The listing builds one solid part. Answer for the finished solid, in the listing's coordinates (mm). Face numbers are marked on the shaded views. A direction names the side the tool comes from. Give positions to 0.01 mm unless a question says otherwise; leave off trailing zeros. Order: outer loops, then holes, each group sorted by start corner. A loop starts at its lowest first (then second) coordinate and runs counter-clockwise, first axis right, second up. Notation, with made-up numbers: (79, 76) - (93, 76) arc R11 ccw to (93, 97) - close; hole circle Ø2 at (-3.75, 59.25). An arc over 180 degrees is marked (long way). Answer in a Markdown table with one row per item.
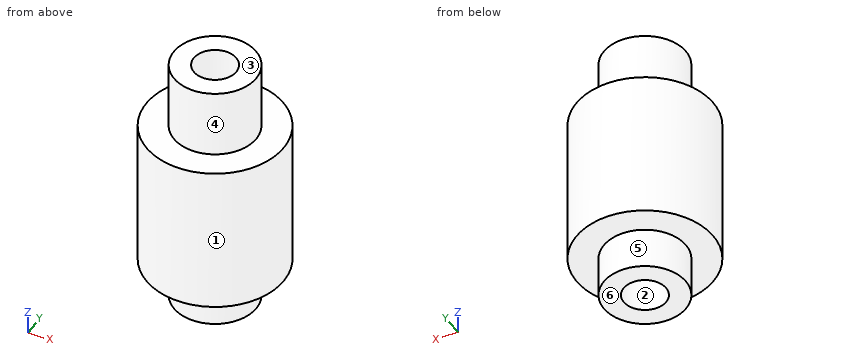
Autodesk Inventor part; units mm, degrees
ref_plane "YZ Plane" through (0, 0, 0) normal (1, 0, 0) x (0, 1, 0)
ref_plane "XZ Plane" through (0, 0, 0) normal (0, 1, 0) x (-1, 0, 0)
ref_plane "XY Plane" through (0, 0, 0) normal (0, 0, 1) x (1, 0, 0)
sketch "スケッチ1" plane through (0, 0, 0) normal (1, 0, 0) x (0, 1, 0)
  line L0 (0, 0) -> (3, 0)
  line L1 (3, 0) -> (3, 5)
  line L2 (3, 5) -> (0, 5)
  line L3 (0, 5) -> (0, 0)
  line L4 (0, 0) -> (5, 0)
  line L5 (5, 0) -> (5, -11)
  line L6 (5, -11) -> (0, -11)
  line L7 (0, -11) -> (0, 0)
  line L8 (0, -11) -> (3, -11)
  line L9 (3, -11) -> (3, -14)
  line L10 (3, -14) -> (0, -14)
  line L11 (0, -14) -> (0, -11)
  dimension "d0" = 3
  dimension "d1" = 5
  dimension "d2" = 5
  dimension "d3" = 11
  dimension "d4" = 3
  dimension "d5" = 3
revolve "回転1" add sketch "スケッチ1" angle 360 about axis through (0, 0, -11) along (0, 0, 1)
sketch "スケッチ2" plane through (0, 0, 5) normal (0, 0, 1) x (1, 0, 0)
  point P0 (0, 0)
  point P1 (0, 0)
hole "穴1" at (0, 0, 5) direction (0, 0, -1) diameter 3.1 end through all
properties part number "ベース板連結棒" material "アルミニウム 6061"
Item 1: Which of the six approach directions +Z, -Z, +X, -X, +Y, -Y give full straight-line access (tool end or side, diameter ignored) to the marked faces 4, 5 and 6?
Answer block:
| item | result |
|---|---|
| face 4 | +Z |
| face 5 | -Z |
| face 6 | -Z, +X, -X, +Y, -Y |
Item 2: Consider line 1 (Y direction, x = 0, z = -4.5); line 2 (Z direction, x = 4.75, y = -0.75). Determine where each line is inside the solid, lowest interval first.
Answer block:
| item | result |
|---|---|
| line 1 | -5 to -1.55, 1.55 to 5 |
| line 2 | -11 to 0 |
Item 3: This flat-tipped pin is pushed along its axis until it touches: P1, Ø1.5, axis at y = -1, z = -1.5, coming from the +X side. Where does it stop, or does it pass through?
Answer block:
| item | result |
|---|---|
| P1 | x = 4.99 |
Item 4: Determine the mould class of the marked faces 1, 2 and 3 for opening direction Y: pulls with the +Y half, pulls with the -Y half, needs draft (parallel to the pull), parting line crosses it, or undercut.
Answer block:
| item | result |
|---|---|
| face 1 | parting line crosses it |
| face 2 | undercut |
| face 3 | needs draft |
Item 5: Find section D-D on z = -10. Write down the section's boundary in (x, y).
Answer block:
| item | result |
|---|---|
| outline | circle Ø10 at (0, 0); hole circle Ø3.1 at (0, 0) |
Item 6: Find section C-C on x = 2. Write down the section's boundary in (y, z).
Answer block:
| item | result |
|---|---|
| outline | (-4.58, -11) - (-2.24, -11) - (-2.24, -14) - (2.24, -14) - (2.24, -11) - (4.58, -11) - (4.58, 0) - (2.24, 0) - (2.24, 5) - (-2.24, 5) - (-2.24, 0) - (-4.58, 0) - close |
Item 7: Find section A-A on y = 0. Write down the section's boundary in (x, z).
Answer block:
| item | result |
|---|---|
| outline | (-5, -11) - (-3, -11) - (-3, -14) - (-1.55, -14) - (-1.55, 5) - (-3, 5) - (-3, 0) - (-5, 0) - close; (1.55, -14) - (3, -14) - (3, -11) - (5, -11) - (5, 0) - (3, 0) - (3, 5) - (1.55, 5) - close |
